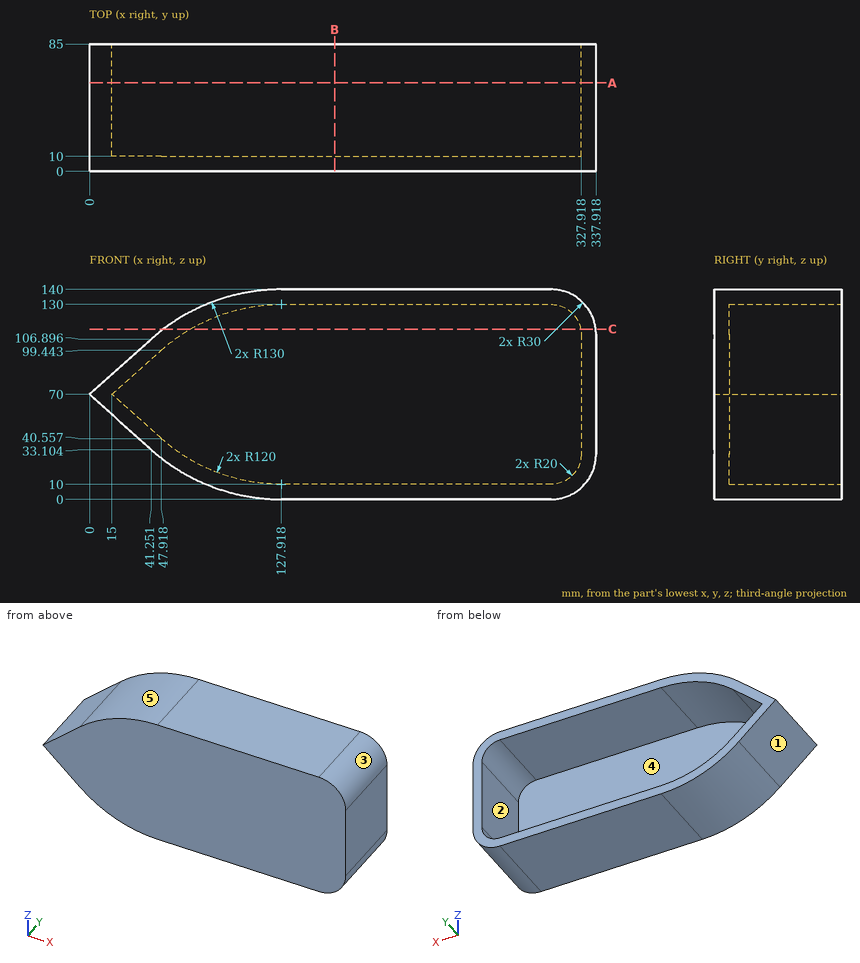
Geometry: see drawing. Coordinates: mm, zero at the bounding-box minimum. A direction names the side the tool comes from. Give positions to 0.01 mm unless a question says otherwise; leave off trailing zeros. Write each loop counter-clockwise with the first axis right and the second up, starting at its lowest first coordinate (ties: lowest second). Pieces come first, ordered by that corner, then holes. Notation, with made-up numbers: M -4,6 L 8,6 A21 ccw 8,25 Z; hole C 47.25,2 d10. An arc over 180 degrees is marked long. Return JSON: item names as keys, results as strings. Group by question number.
1) Cut plane A-A, the plane y = 59. Output: boundary loops of the cut face in (x, z).
2) First-contact query: pin 1 Ø8 at (y, z) = (68.5, 97.5) entering from -X (1 decimal). Flat tip, straight axial feed; report the tip coordinate or a pass-through.
3) Draft query along X for the marked faces 3, 4 and 5. Return one class per face: released by +X, released by -X, zero draft, split by the parting line, or undercut.
4) Set-up query: the marked faces 1 and 2. Return all of +Z, -Z, +X, -X, +Y, -Y with unobstructed straight access to the full face (end or side cutting, diameter ignored); none if empty.
5) Cut plane C-C, the plane z = 113.5. Output: boundary loops of the cut face in (x, y), then the cut area to 3 significant figures.
6) Cut plane B-B, the plane x = 163.5. Output: boundary loops of the cut face in (y, z), then the cut area to 3 significant figures.
7) Ray query, L1, parallel to Z at x = 191.5, y = 50; L2, parallel to Y at x = 309, z = 22; L3, parallel to Z at x = 104, y = 27.5. Return the intervals inside material, ascending.
Data:
{
 "1": {"outline": "M 0,70 L 41.25,33.1 A130 ccw 127.92,0 L 307.92,0 A30 ccw 337.92,30 L 337.92,110 A30 ccw 307.92,140 L 127.92,140 A130 ccw 41.25,106.9 Z; hole M 15,70 L 47.92,40.56 A120 ccw 127.92,10 L 307.92,10 A20 ccw 327.92,30 L 327.92,110 A20 ccw 307.92,130 L 127.92,130 A120 ccw 47.92,99.44 Z"},
 "2": {"pin 1": "stops at x = 26.3"},
 "3": {"face 3": "released by +X", "face 4": "undercut", "face 5": "released by -X"},
 "4": {"face 1": "-Z, -X, +Y, -Y", "face 2": "+Y"},
 "5": {"outline": "M 49.26,0 L 337.71,0 L 337.71,85 L 327.61,85 L 327.61,10 L 67.19,10 L 67.19,85 L 49.26,85 Z", "area": "4,990 mm²"},
 "6": {"outline": "M 0,0 L 85,0 L 85,10 L 10,10 L 10,130 L 85,130 L 85,140 L 0,140 Z", "area": "2,900 mm²"},
 "7": {"L1": "z = 0 to 10, 130 to 140", "L2": "y = 0 to 10", "L3": "z = 2.22 to 12.41, 127.59 to 137.78"}
}
